Geometry check sheet. Reference: drawing and pictorial views, mm from the part's lowest x, y, z. Give positions to 0.01 mm unless a question says otherwise; leave off trailing zeros. Order: outer loops, then holes, each group sorted by start corner. A loop starts at its lowest first (then second) coordinate and runs counter-clockwise, first axis right, second up. Notation, with made-up numbers: M 45,-25 L 66,-25 A24 ccw 66,13 Z; hole C -11,-10.5 d4. An arc over 180 degrees is marked long. Answer as a JSON object with one key per item and string values. Group by question number.
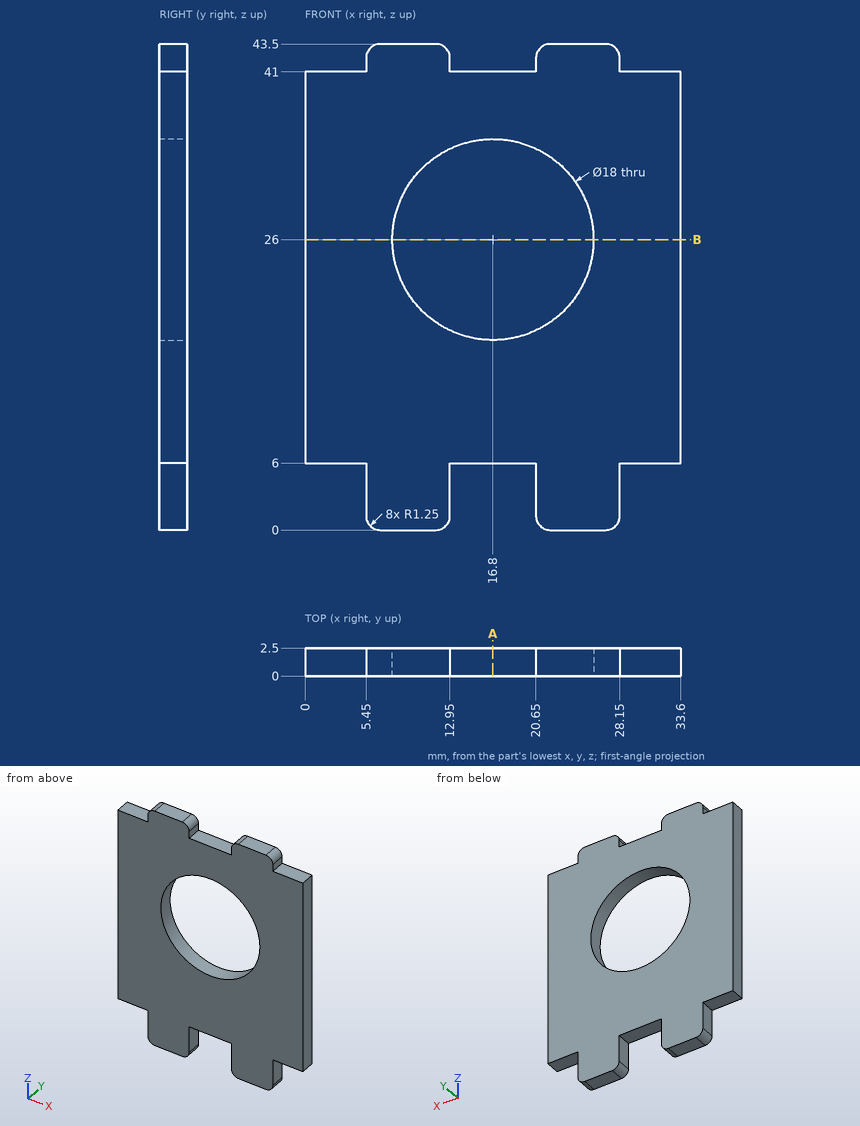
1. Depth check by flat-ended pin: pin 1 (1.5 mm diameter, centred on x = 6, y = 2, fed in from +Z); pin 2 (1.2 mm diameter, centred on y = 1.5, z = 3.5, fed in from -X); pin 3 (1.4 mm diameter, centred on y = 1.5, z = 42, fed in from -X); pin 4 (3 mm diameter, centred on x = 21.5, z = 30.5, fed in from -Y). Enter the tip coordinate at first touch or a pass-through.
2. Cross-section at B-B (z = 26). Record the cut outline in (x, y).
3. Cross-section at A-A (x = 16.8). Record the cut outline in (y, z).
4. Thickness scan on line 1 along X through (y, z) = (0.5, 26); line 2 along Z through (x, y) = (16.8, 1.55); line 3 along X through (y, z) = (2.2, 3.5). Record the ranges inside material, lowest first. Write a range as [from, to].
Report:
{
 "1": {"pin 1": "stops at z = 43.5", "pin 2": "stops at x = 5.45", "pin 3": "stops at x = 5.45", "pin 4": "passes through"},
 "2": {"outline": "M 0,0 L 7.8,0 L 7.8,2.5 L 0,2.5 Z; M 25.8,0 L 33.6,0 L 33.6,2.5 L 25.8,2.5 Z"},
 "3": {"outline": "M 0,6 L 2.5,6 L 2.5,17 L 0,17 Z; M 0,35 L 2.5,35 L 2.5,41 L 0,41 Z"},
 "4": {"line 1": "x = [0, 7.8], [25.8, 33.6]", "line 2": "z = [6, 17], [35, 41]", "line 3": "x = [5.45, 12.95], [20.65, 28.15]"}
}
